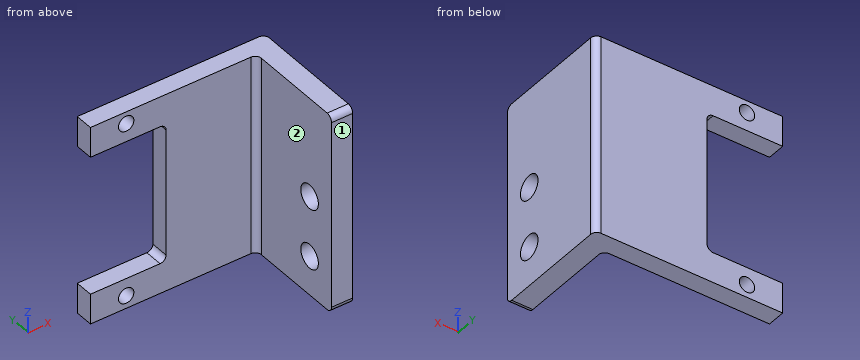
```python
from build123d import *

# Parameters (mm, degrees)
SKETCH1_W             = 15
SKETCH1_H             = 5
SKETCH1_R             = 1.27
BOSS_EXTRUDE1_DEPTH   = 3
BOSS_EXTRUDE1_2_DEPTH = 3
SKETCH2_W             = 2.5
SKETCH2_H             = 28
SKETCH2_H_2           = 5
BOSS_EXTRUDE2_DEPTH   = 20
SKETCH3_W             = 15
SKETCH3_H             = 17
CUT_EXTRUDE1_DEPTH    = 34
SKETCH4_R             = 2
CUT_EXTRUDE2_DEPTH    = 4.5
FILLET1_R             = 1


with BuildPart() as part:
    # Sketch1 → Boss-Extrude1 (new body)
    with BuildSketch(Plane(origin=(0, -5.173201946, 0), x_dir=(1, 0, 0), z_dir=(0, 1, 0))):
        with Locations((7.5, -2.5)):
            Rectangle(SKETCH1_W, SKETCH1_H)
        with Locations((5.906433977, -2.119480538)):
            Circle(SKETCH1_R, mode=Mode.SUBTRACT)
    extrude(amount=BOSS_EXTRUDE1_DEPTH)



with BuildPart() as body_2:
    # Sketch1 → Boss-Extrude1 2 (new body)
    with BuildSketch(Plane(origin=(0, -5.173201946, 0), x_dir=(1, 0, 0), z_dir=(0, 1, 0))):
        with Locations((7.5, -30.5)):
            Rectangle(SKETCH1_W, SKETCH1_H)
        with Locations((5.906433977, -31.007519462)):
            Circle(SKETCH1_R, mode=Mode.SUBTRACT)
    extrude(amount=BOSS_EXTRUDE1_2_DEPTH)


with BuildPart() as part_1:
    add(part.part)

    add(body_2.part)  # Boss-Extrude2 merges body 2
    # Sketch2 → Boss-Extrude2 (add)
    with BuildSketch(Plane(origin=(0, -2.173201946, 0), x_dir=(1, 0, 0), z_dir=(0, 1, 0))):
        with Locations((13.75, -14)):
            Rectangle(SKETCH2_W, SKETCH2_H)
        Polygon((31, 0), (15, 0), (15, -28), (15, -33), (31, -33), align=None)
        with Locations((13.75, -30.5)):
            Rectangle(SKETCH2_W, SKETCH2_H_2)
    extrude(amount=-BOSS_EXTRUDE2_DEPTH)

    # Sketch3 → Cut-Extrude1 (cut, through all)
    with BuildSketch(Plane(origin=(0, 0, 0), x_dir=(-1, 0, 0), z_dir=(0, 0, -1))):
        with Locations((-20, -13.673201946)):
            Rectangle(SKETCH3_W, SKETCH3_H)
    extrude(amount=-CUT_EXTRUDE1_DEPTH, mode=Mode.SUBTRACT)

    # Sketch4 → Cut-Extrude2 (cut, through all)
    with BuildSketch(Plane.ZY.offset(-27.5)):
        with Locations((16.5, -17.173201946)):
            Circle(SKETCH4_R)
        with Locations((6.5, -17.173201946)):
            Circle(SKETCH4_R)
    extrude(amount=-CUT_EXTRUDE2_DEPTH, mode=Mode.SUBTRACT)

    # Fillet1
    fillet1_edges = [part_1.edges().sort_by_distance(p)[0] for p in [
        (12.5, -3.673201946, 5),
        (31, -2.173201946, 16.5),
        (12.5, -3.673201946, 28),
        (29.25, -22.173201946, 33),
        (29.25, -22.173201946, 0),
        (27.5, -5.173201946, 16.5),
    ]]
    fillet(fillet1_edges, radius=FILLET1_R)


solid = part_1.part
```
Can you work these out from the model? Positions are in its coordinate system, mm. Face numbers are marked on the shaded views. A direction names the side the tool comes from. Round coordinates to 2 decimals unless told otherwise and drop trailing zeros. Loops run counter-clockwise (first coordinate to the right, second up) from the corner with the lowest first, then second, coordinate; pieces in that order, holes last. Notation, with made-up numbers: (60, 68) -> (92, 68) arc R14 cw to (92, 91) -> close; hole circle Ø4 at (63.5, -24). An arc over 180 degrees is marked (long way). Answer in a Markdown table with one row per item.
Item 1: Suppose I cut it at C-C, the plane y = -16.25. List the corners of the cut face in (x, z) for me.
Answer block:
| item | result |
|---|---|
| outline | (27.5, 0) -> (31, 0) -> (31, 4.73) -> (27.5, 4.73) -> close; (27.5, 8.27) -> (31, 8.27) -> (31, 14.73) -> (27.5, 14.73) -> close; (27.5, 18.27) -> (31, 18.27) -> (31, 33) -> (27.5, 33) -> close |
Item 2: Suppose I cut it at D-D, the plane z = 21. List the corners of the cut face in (x, y) for me.
Answer block:
| item | result |
|---|---|
| outline | (12.5, -5.17) -> (26.5, -5.17) arc R1 cw to (27.5, -6.17) -> (27.5, -22.17) -> (31, -22.17) -> (31, -3.17) arc R1 ccw to (30, -2.17) -> (12.5, -2.17) -> close |
Item 3: If I drill on probe 1 along Y at (x, z) = (29.65, 16.5); probe 2 along Y at (x, z) = (25, 7.5); probe 3 along X at (y, z) = (-14.5, 23.5), over which ranges is the centre line in solid material (lowest first)?
Answer block:
| item | result |
|---|---|
| probe 1 | -22.17 to -19.17, -15.17 to -2.17 |
| probe 2 | -5.17 to -2.17 |
| probe 3 | 27.5 to 31 |
Item 4: Suppose I cut it at A-A, the plane x = 11. List the corners of the cut face in (y, z) for me, plus the area to 3 significant figures.
Answer block:
| item | result |
|---|---|
| outline | (-5.17, 0) -> (-2.17, 0) -> (-2.17, 5) -> (-5.17, 5) -> close; (-5.17, 28) -> (-2.17, 28) -> (-2.17, 33) -> (-5.17, 33) -> close |
| area | 30.0 mm² |
Item 5: Suppose I cut it at B-B, the plane z = 16.5. List the corners of the cut face in (x, y) for me.
Answer block:
| item | result |
|---|---|
| outline | (12.5, -5.17) -> (26.5, -5.17) arc R1 cw to (27.5, -6.17) -> (27.5, -15.17) -> (31, -15.17) -> (31, -3.17) arc R1 ccw to (30, -2.17) -> (12.5, -2.17) -> close; (27.5, -22.17) -> (31, -22.17) -> (31, -19.17) -> (27.5, -19.17) -> close |
Item 6: Will these pins go through, and if not, where does the flat tip stop? P1, Ø8, axis at x = 22, z = 26.5, coming from the -Y side; P2, Ø1.5, axis at x = 5.91, z = 2.12, coming from the -Y side; P3, Ø6.5, axis at y = -17.17, z = 16.5, coming from the -X side; P4, Ø2.5, axis at y = -4, z = 20.5, coming from the -X side.
Answer block:
| item | result |
|---|---|
| P1 | y = -5.17 |
| P2 | through |
| P3 | x = 27.5 |
| P4 | x = 12.5 |
Item 7: On a 3-axis mill with a long thin cutter (end or side, diameter ignored), from which of +Z, -Z, +X, -X, +Y, -Y can I reach the whole of each face in a straight line? I mean the marked faces 1 and 2. Say none if no direction works.
Answer block:
| item | result |
|---|---|
| face 1 | +Z, -Z, +X, -X, -Y |
| face 2 | +Z, -Z, -X, -Y |
